Read the model definition and answer for the solid it produces. Units are mm, in the model's axes. Round coordinates to 2 decimals unless told otherwise and drop trailing zeros. Write each loop counter-clockwise with the first axis right and the second up, starting at its lowest first coordinate (ties: lowest second). Pieces come first, ordered by that corner, then holes.
from build123d import *

# Parameters (mm, degrees)
CYLINDER001_R     = 4
CYLINDER001_DEPTH = 15
CYLINDER_R        = 5
CYLINDER_DEPTH    = 15


with BuildPart() as con001:
    # Cone001 → Cone001 (revolve)
    with BuildSketch(Plane(origin=(0, 0, 15), x_dir=(1, 0, 0), z_dir=(0, -1, 0))):
        Polygon((0, 0), (4, 0), (24, 30), (0, 30), align=None)
    revolve(axis=Axis((0, 0, 15), (0, 0, 1)))


with BuildPart() as cut001:
    # Cone → Cone (revolve)
    with BuildSketch(Plane(origin=(0, 0, 15), x_dir=(1, 0, 0), z_dir=(0, -1, 0))):
        Polygon((0, 0), (5, 0), (25, 30), (0, 30), align=None)
    revolve(axis=Axis((0, 0, 15), (0, 0, 1)))

    # Cut001: cut Con001
    add(con001.part, mode=Mode.SUBTRACT)


with BuildPart() as cilindre001:
    # Cylinder001 → Cylinder001 (new body)
    with BuildSketch(Plane.XY):
        Circle(CYLINDER001_R)
    extrude(amount=CYLINDER001_DEPTH)


with BuildPart() as fusion:
    # Cylinder → Cylinder (new body)
    with BuildSketch(Plane.XY):
        Circle(CYLINDER_R)
    extrude(amount=CYLINDER_DEPTH)

    # Cut: cut Cilindre001
    add(cilindre001.part, mode=Mode.SUBTRACT)

    # Fusion: union Cut001
    add(cut001.part)


solid = fusion.part
Q1. Flat-ended cylindrical pins translate along their axes: pin 1 Ø4 at (x, z) = (-6.5, 16.5) entering from +Y; pin 2 Ø1.5 at (x, z) = (-2, 34) entering from -Y; pin 3 Ø8 at (x, z) = (-6.5, 6) entering from -Y. Find the tip coordinate at first contact, or state that the pin passes through.
Verdict:
pin 1: stops at y = 4.73
pin 2: stops at y = -18.06
pin 3: stops at y = -4.33
Q2. Section A-A (x = 0) is taken. Determine the outline of the cut face in (y, z).
Verdict:
outline: (-25, 45) - (-5, 15) - (-5, 0) - (-4, 0) - (-4, 15) - (-24, 45) - close; (4, 0) - (5, 0) - (5, 15) - (25, 45) - (24, 45) - (4, 15) - close
Q3. Determine the mould class of faces 1 (the cylindrical face through (-0.867, -3.905, 7.395)), 2 (the cylindrical face through (-1.08, -4.88, 7.4)), 3 (the flat face through (-9.4, 22.3, 45)) for opening direction X: pulls with the +X half, pulls with the -X half, needs draft (parallel to the pull), parting line crosses it, or undercut.
Verdict:
face 1: undercut
face 2: parting line crosses it
face 3: needs draft
Q4. Section D-D (z = 27) is taken. Determine the outline of the cut face in (x, y).
Verdict:
outline: circle Ø26 at (0, 0); hole circle Ø24 at (0, 0)
Q5. Straight lines are drawn through the part: probe 1 along Y at (x, z) = (0, 10.5); probe 2 along X at (y, z) = (-4, 24); probe 3 along X at (y, z) = (3, 14). For each, find the intervals that lie inside material, in ascending order.
Verdict:
probe 1: y = -5 to -4, 4 to 5
probe 2: x = -10.25 to -9.17, 9.17 to 10.25
probe 3: x = -4 to -2.65, 2.65 to 4
Q6. Section C-C (z = 7.5) is taken. Determine the outline of the cut face in (x, y), then the cut area to 3 significant figures.
Verdict:
outline: circle Ø10 at (0, 0); hole circle Ø8 at (0, 0)
area: 28.3 mm2
